The listing builds one solid part. Answer for the finished solid, in the listing's coordinates (mm). Coordinates: 2 decimals unless noted, no trailing zeros. Loops run counter-clockwise (first coordinate to the right, second up) from the corner with the lowest first, then second, coordinate; pieces in that order, holes last. Notation, with made-up numbers: (-2.75, -19.75) - (40.25, -19.75) arc R28 ccw to (40.25, 16.25) - close; hole circle Ø1 at (-27.75, -28.5). An arc over 180 degrees is marked (long way). Return JSON: item names as keys, results as strings. Group by question number.
1. Each of these flat-tipped pins is pushed along its axis until it touches: P1, Ø1.5, axis at y = 8, z = -4, coming from the -X side; P2, Ø1.6, axis at x = 68, y = 7, coming from the -Z side (3 decimals); P3, Ø1.5, axis at y = 30.5, z = -2.5, coming from the +X side. Where does it stop, or does it pass through?
2. Section A-A (z = -4.75) is taken. State how many separate pieces and enclosed holes the cut face has, and give its area (3 significant figures).
3. Section C-C (y = 23.5) is taken. Write down the section's boundary in (x, z), and give its area (3 significant figures).
4. Find the intervals of material crossed by line 1 along Z through (x, y) = (53.5, 45) (3 decimals); line 2 along X through (y, z) = (14, -5.75); line 3 along X through (y, z) = (53, -4), in increasing order.
```python
from build123d import *

# Parameters (mm, degrees)
SKETCH1_W           = 152.4
SKETCH1_H           = 57.15
BOSS_EXTRUDE1_DEPTH = 6.35
CUT_EXTRUDE2_DEPTH  = 58.15
SKETCH4_W           = 3.175
SKETCH4_H           = 4.7625
CUT_EXTRUDE3_DEPTH  = 153.4
SKETCH5_W           = 3.175
SKETCH5_H           = 3.2512
CUT_EXTRUDE4_DEPTH  = 153.4
SKETCH6_R           = 2.38125
CUT_EXTRUDE5_DEPTH  = 5.08


with BuildPart() as part:
    # Sketch1 → Boss-Extrude1 (new body)
    with BuildSketch(Plane.XY):
        with Locations((76.2, 28.575)):
            Rectangle(SKETCH1_W, SKETCH1_H)
    extrude(amount=-BOSS_EXTRUDE1_DEPTH)

    # Sketch3 → Cut-Extrude2 (cut, through all)
    with BuildSketch(Plane(origin=(0, 57.15, 0), x_dir=(1, 0, 0), z_dir=(0, 1, 0))):
        Polygon((152.4, 0), (146.05, 6.35), (152.4, 6.35), align=None)
        Polygon((0, 0), (6.35, 6.35), (0, 6.35), align=None)
    extrude(amount=-CUT_EXTRUDE2_DEPTH, mode=Mode.SUBTRACT)

    # Sketch4 → Cut-Extrude3 (cut, through all)
    with BuildSketch(Plane(origin=(0, 0, 0), x_dir=(0, 0, -1), z_dir=(1, 0, 0))):
        with Locations((4.7625, 43.97375)):
            Rectangle(SKETCH4_W, SKETCH4_H)
    extrude(amount=CUT_EXTRUDE3_DEPTH, mode=Mode.SUBTRACT)

    # Sketch5 → Cut-Extrude4 (cut, through all)
    with BuildSketch(Plane(origin=(0, 0, 0), x_dir=(0, 0, -1), z_dir=(1, 0, 0))):
        with Locations((4.7625, 6.3881)):
            Rectangle(SKETCH5_W, SKETCH5_H)
    extrude(amount=CUT_EXTRUDE4_DEPTH, mode=Mode.SUBTRACT)

    # Sketch6 → Cut-Extrude5 (cut)
    with BuildSketch(Plane(origin=(0, 0, -6.35), x_dir=(-1, 0, 0), z_dir=(0, 0, -1))):
        with Locations((-142.748, 49.911)):
            Circle(SKETCH6_R)
    extrude(amount=-CUT_EXTRUDE5_DEPTH, mode=Mode.SUBTRACT)


solid = part.part
```
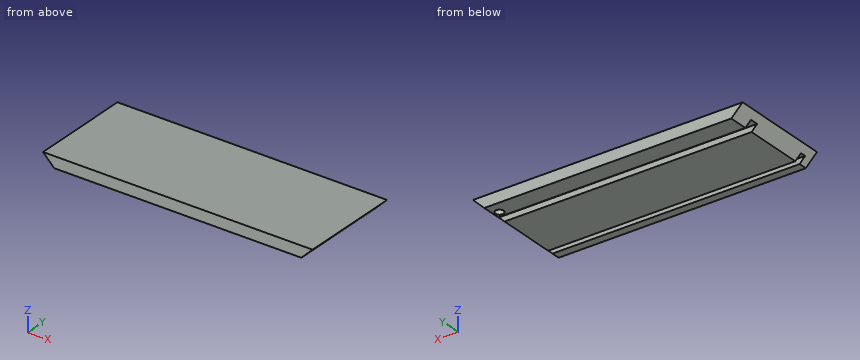
The answers:
{
 "1": {"P1": "stops at x = 3.25", "P2": "stops at z = -3.175", "P3": "stops at x = 150.65"},
 "2": {"separate pieces": "3", "enclosed holes": "1", "area": "7,000 mm2"},
 "3": {"outline": "(0, 0) - (6.35, -6.35) - (146.05, -6.35) - (152.4, 0) - close", "area": "927 mm2"},
 "4": {"line 1": "z = -3.175 to 0", "line 2": "x = 5.75 to 146.65", "line 3": "x = 4 to 148.4"}
}
